For this review, take the finished solid that the model builds, in its own axes (mm). A direction names the side the tool comes from. Round coordinates to 2 decimals unless told otherwise and drop trailing zeros. Write each loop counter-clockwise with the first axis right and the second up, starting at its lowest first coordinate (ties: lowest second). Pieces come first, ordered by that corner, then holes. Notation, with made-up numbers: M 29.25,37 L 84.25,37 A17 ccw 84.25,59 Z; hole C 74,33.25 d1. An arc over 180 degrees is marked long. Answer in a Markdown table with one row per item.
```python
from build123d import *

# Parameters (mm, degrees)
SKETCH1_W           = 87.47
SKETCH1_H           = 60.6
BOSS_EXTRUDE1_DEPTH = 3.175
BOSS_EXTRUDE2_DEPTH = 3.175
FILLET1_R           = 5
SKETCH5_R           = 1.415
CUT_EXTRUDE2_DEPTH  = 10
SKETCH6_W           = 87.47
SKETCH6_H           = 3.265
CUT_EXTRUDE3_DEPTH  = 10
SKETCH2_W           = 30.83
SKETCH2_H           = 22.08
SKETCH2_W_2         = 31.83
CUT_EXTRUDE4_DEPTH  = 10
SKETCH8_W           = 87.47
SKETCH8_H           = 0.09
BOSS_EXTRUDE3_DEPTH = 3.175


with BuildPart() as part:
    # Sketch1 → Boss-Extrude1 (new body)
    with BuildSketch(Plane.XY):
        Rectangle(SKETCH1_W, SKETCH1_H)
    extrude(amount=BOSS_EXTRUDE1_DEPTH)

    # Sketch3 → Boss-Extrude2 (add)
    with BuildSketch(Plane.XY.offset(3.175)):
        with BuildLine():
            Line((43.735, 10.085), (43.735, -10.085))
            Line((43.735, -10.085), (73.735, -10.085))
            ThreePointArc((73.735, -10.085), (83.82, 0), (73.735, 10.085))
            Line((73.735, 10.085), (43.735, 10.085))
        make_face()
    extrude(amount=-BOSS_EXTRUDE2_DEPTH)

    # Fillet1
    fillet1_edges = [part.edges().sort_by_distance(p)[0] for p in [
        (43.735, -10.085, 1.5875),
        (43.735, 10.085, 1.5875),
    ]]
    fillet(fillet1_edges, radius=FILLET1_R)

    # Sketch5 → Cut-Extrude2 (cut)
    with BuildSketch(Plane.XY.offset(3.175)):
        with Locations((73.735, 0)):
            Circle(SKETCH5_R)
    extrude(amount=-CUT_EXTRUDE2_DEPTH, mode=Mode.SUBTRACT)

    # Sketch6 → Cut-Extrude3 (cut)
    with BuildSketch(Plane.XY.offset(3.175)):
        with Locations((0, 28.6675)):
            Rectangle(SKETCH6_W, SKETCH6_H)
        with Locations((0, -28.6675)):
            Rectangle(SKETCH6_W, SKETCH6_H)
    extrude(amount=-CUT_EXTRUDE3_DEPTH, mode=Mode.SUBTRACT)

    # Sketch2 → Cut-Extrude4 (cut)
    with BuildSketch(Plane.XY.offset(3.175)):
        with Locations((20.25, 14.675)):
            Rectangle(SKETCH2_W, SKETCH2_H)
        with Locations((-20.25, 14.675)):
            Rectangle(SKETCH2_W, SKETCH2_H)
        with Locations((0, -14.675)):
            Rectangle(SKETCH2_W_2, SKETCH2_H)
    extrude(amount=-CUT_EXTRUDE4_DEPTH, mode=Mode.SUBTRACT)

    # Sketch8 → Boss-Extrude3 (add)
    with BuildSketch(Plane.XY.offset(3.175)):
        with Locations((0, 27.08)):
            Rectangle(SKETCH8_W, SKETCH8_H)
        with Locations((0, -27.08)):
            Rectangle(SKETCH8_W, SKETCH8_H)
    extrude(amount=-BOSS_EXTRUDE3_DEPTH)


solid = part.part
```
Q1. Take a section at D-D (z = 1.8). State the section outline as (x, y) points (3 decimals).
Found:
| item | result |
|---|---|
| outline | M -43.735,-27.125 L 43.735,-27.125 L 43.735,-15.085 A5 cw 48.735,-10.085 L 73.735,-10.085 A10.085 ccw 73.735,10.085 L 48.735,10.085 A5 cw 43.735,15.085 L 43.735,27.125 L -43.735,27.125 Z; hole M -35.665,3.635 L -4.835,3.635 L -4.835,25.715 L -35.665,25.715 Z; hole M -15.915,-25.715 L 15.915,-25.715 L 15.915,-3.635 L -15.915,-3.635 Z; hole M 4.835,3.635 L 35.665,3.635 L 35.665,25.715 L 4.835,25.715 Z; hole C 73.735,0 d2.83 |
Q2. Take a section at B-B (y = 0). State the section outline as (x, z) points (3 decimals).
Found:
| item | result |
|---|---|
| outline | M -43.735,0 L 72.32,0 L 72.32,3.175 L -43.735,3.175 Z; M 75.15,0 L 83.82,0 L 83.82,3.175 L 75.15,3.175 Z |
Q3. Take a section at A-A (x = -9). State the section outline as (y, z) points (3 decimals).
Found:
| item | result |
|---|---|
| outline | M -27.125,0 L -25.715,0 L -25.715,3.175 L -27.125,3.175 Z; M -3.635,0 L 3.635,0 L 3.635,3.175 L -3.635,3.175 Z; M 25.715,0 L 27.125,0 L 27.125,3.175 L 25.715,3.175 Z |
Q4. Insertion check: P1, Ø1, axis at x = 64, z = 1, coming from the -Y side (3 decimals); P2, Ø5, axis at x = 25, y = -16.5, coming from the -Z side. Each pin has a flat end and moves straight along its axis. Give the tip position at first contact, or say it passes through.
Found:
| item | result |
|---|---|
| P1 | y = -10.085 |
| P2 | z = 0 |
Q5. For probe 1 along X at (y, z) = (24, 0.9) (3 decimals); probe 2 along Y at (x, z) = (-12, 2.1) (3 decimals); probe 3 along Y at (x, z) = (20, 2.5) (3 decimals), list the stretches that pass through material, from the lowest coordinate up.
Found:
| item | result |
|---|---|
| probe 1 | -43.735 to -35.665, -4.835 to 4.835, 35.665 to 43.735 |
| probe 2 | -27.125 to -25.715, -3.635 to 3.635, 25.715 to 27.125 |
| probe 3 | -27.125 to 3.635, 25.715 to 27.125 |
Q6. Take a section at C-C (y = 19.5). State the section outline as (x, z) points (3 decimals).
Found:
| item | result |
|---|---|
| outline | M -43.735,0 L -35.665,0 L -35.665,3.175 L -43.735,3.175 Z; M -4.835,0 L 4.835,0 L 4.835,3.175 L -4.835,3.175 Z; M 35.665,0 L 43.735,0 L 43.735,3.175 L 35.665,3.175 Z |
Q7. Mouldability with a two-part tool opening along X and no side actions: class faces 1 (the face through (83.818, -0.222, 1.61)), 2 (the face through (35.665, 15, 2)), 3 (the face through (-1, -27.125, 2)) as +X half, -X half, draft (parallel to the pull), parting line (faces both ways), or undercut.
Found:
| item | result |
|---|---|
| face 1 | +X half |
| face 2 | undercut |
| face 3 | draft |
Q8. Machinability: for faces 4 (the face through (-15.915, -15, 2)), 5 (the face through (43.735, 21, 2)), 6 (the face through (5, 0, 3.175)), 7 (the face through (61, -10.085, 2)), which of the approach directions +Z, -Z, +X, -X, +Y, -Y give a long, thin tool a straight path to every point of the face, cutting with its end or side? Answer none if there is none.
Found:
| item | result |
|---|---|
| face 4 | +Z, -Z |
| face 5 | +Z, -Z, +X, +Y |
| face 6 | +Z, +X, -X, +Y, -Y |
| face 7 | +Z, -Z, +X, -Y |
